The figure shows three views and two pictorial views of one solid part (mm, origin at its lowest corner). Answer the questions. Coordinates: 2 decimals unless noted, no trailing zeros. Loops run counter-clockwise (first coordinate to the right, second up) from the corner with the lowest first, then second, coordinate; pieces in that order, holes last. Notation, with made-up numbers: M 7,78.5 L 43,78.5 A15 ccw 43,104.5 Z; hole C -5,3.25 d10. An arc over 180 degrees is marked long. Write each question's results on one line, items separated by ' | '.
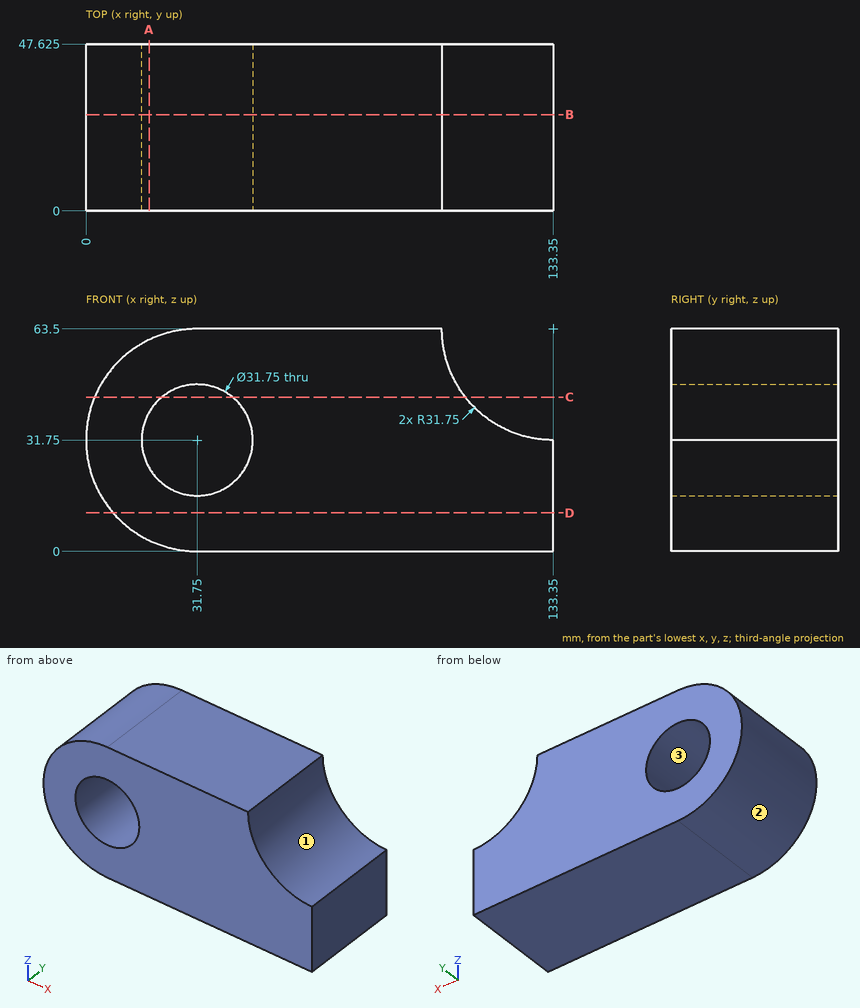
1) Find section A-A, the plane x = 18. Give the vertices of the cut face in (y, z) (3 decimals), and give its area (3 significant figures).
Check result:
outline: M 0,3.132 L 47.625,3.132 L 47.625,23.816 L 0,23.816 Z; M 0,39.684 L 47.625,39.684 L 47.625,60.368 L 0,60.368 Z | area: 1,970 mm^2
2) Find section D-D, the plane z = 11. Give the vertices of the cut face in (x, y) (3 decimals), and give its area (3 significant figures).
Check result:
outline: M 7.719,0 L 133.35,0 L 133.35,47.625 L 7.719,47.625 Z | area: 5,980 mm^2
3) Find section B-B, the plane y = 27.5. Give the vertices of the cut face in (x, z) (3 decimals).
Check result:
outline: M 31.75,0 L 133.35,0 L 133.35,31.75 A31.75 cw 101.6,63.5 L 31.75,63.5 A31.75 ccw Z; hole C 31.75,31.75 d31.75
4) Given pin 1 Ø4 at (x, y) = (20, 29.5) entering from -Z; pin 2 Ø3 at (y, z) = (24, 22.5) entering from -X; pin 3 Ø3 at (y, z) = (22, 45.5) entering from -X, each flat-ended and moving along its own axis, determine where each tip first touches the part or whether it passes through.
Check result:
pin 1: z = 1.53 | pin 2: x = 0.96 | pin 3: x = 2.46
5) For a pull along Z with two mould halves and no side action, classify the marked faces 1, 2 and 3 as released by +Z, released by -Z, zero draft, split by the parting line, or undercut.
Check result:
face 1: released by +Z | face 2: split by the parting line | face 3: undercut
6) Straight lines are drawn through the part: probe 1 along X at (y, z) = (37, 31); probe 2 along Z at (x, y) = (32, 32.5); probe 3 along X at (y, z) = (36, 39). For each, find the intervals that lie inside material, in ascending order. Write a range as [from, to].
Check result:
probe 1: [0.01, 15.89], [47.61, 133.35] | probe 2: [0, 15.88], [47.62, 63.5] | probe 3: [0.84, 17.63], [45.87, 113.16]
7) Find section C-C, the plane z = 44. Give the vertices of the cut face in (x, y) (3 decimals).
Check result:
outline: M 2.458,0 L 21.653,0 L 21.653,47.625 L 2.458,47.625 Z; M 41.847,0 L 108.294,0 L 108.294,47.625 L 41.847,47.625 Z
